Verification items for the finished model (mm, model axes). A direction names the side the tool comes from. Round coordinates to 2 decimals unless told otherwise and drop trailing zeros. Write each loop counter-clockwise with the first axis right and the second up, starting at its lowest first coordinate (ties: lowest second). Pieces come first, ordered by that corner, then holes.
Solid Edge part; units mm, degrees
sketch "Sketch1" plane through (0, 0, 0) normal (0, 0, 1) x (1, 0, 0)
  line L0 (0, 0) -> (12.7, 0)
  line L1 (0, 0) -> (-5.8373, 4.898)
sketch "Sketch2" plane through (12.7, 0, 0) normal (1, 0, 0) x (0, 1, 0)
  line L0 (1.5875, -1.5875) -> (1.5875, 1.5875)
  line L1 (1.5875, 1.5875) -> (-1.5875, 1.5875)
  line L2 (-1.5875, 1.5875) -> (-1.5875, -1.5875)
  line L3 (-1.5875, -1.5875) -> (1.5875, -1.5875)
sweep "SweptProtrusion_1" add profiles "Sketch2" path "Sketch1"
sketch "Sketch3" plane through (0, 0, 0) normal (0, 0, 1) x (1, 0, 0)
  line L0 (0, 0) -> (12.7, 0)
  line L1 (0, 0) -> (-6.5307, -7.783)
sketch "Sketch4" plane through (12.7, 0, 0) normal (1, 0, 0) x (0, 1, 0)
  line L0 (-1.5875, -1.5875) -> (1.5875, -1.5875)
  line L1 (1.5875, -1.5875) -> (1.5875, 1.5875)
  line L2 (1.5875, 1.5875) -> (-1.5875, 1.5875)
  line L3 (-1.5875, 1.5875) -> (-1.5875, -1.5875)
sweep "SweptProtrusion_2" add profiles "Sketch4" path "Sketch3"
sketch "Sketch5" plane through (-2.2223, 2.052, 1.5875) normal (0, 0, 1) x (1, 0, 0)
  circle A0 centre (2.2223, -2.052) radius 0.3969
extrude "Cutout1" cut sketch "Sketch5" against normal up to next
fillet "Round_1" radius 0.254 27 edges at (6.7201, -1.5875, 1.5875) (-2.2872, -5.1955, 1.5875) (-4.9917, -3.4791, 1.5875) (-4.5471, 1.7431, 1.5875) (-2.1195, 3.8508, 1.5875) (6.6389, 1.5875, 1.5875) (12.7, 0, 1.5875) (12.7, 0, -1.5875) (12.7, -1.5875, 0) (12.7, 1.5875, 0) (6.7201, -1.5875, -1.5875) (0.7403, -1.5875, 0) (-2.2872, -5.1955, -1.5875) (-6.5307, -7.783, 1.5875) (-5.3146, -8.8034, 0) (-6.5307, -7.783, -1.5875) (-7.7468, -6.7626, 0) (-2.2365, -0.1957, 0) (-4.9917, -3.4791, -1.5875) (-4.5471, 1.7431, -1.5875) (-6.8577, 3.6819, 0) (-5.8373, 4.898, 1.5875) (-4.8168, 6.1141, 0) (-5.8373, 4.898, -1.5875) (0.5778, 1.5875, 0) (6.6389, 1.5875, -1.5875) (-2.1195, 3.8508, -1.5875)
Q1. Tool access check on faces 4 (the cylindrical face through (-4.47, 1.77, -1.51)), 5 (the flat face through (7, 1.588, 0)), 6 (the cylindrical face through (-4.468, 1.777, 1.515)). Record the directions out of +Z, -Z, +X, -X, +Y, -Y that give a thin tool (end or side, any length) a straight path to the whole face; none if there is none.
Recorded:
face 4: -Z, -X
face 5: +Z, -Z, +X, +Y
face 6: +Z, -X
Q2. Sectioned sample at A-A (z = 0.4). Enter the section's corners in (x, y), plus the area to 3 significant figures.
Recorded:
outline: (-7.58, -6.57) arc R0.25 ccw to (-7.55, -6.93) - (-5.51, -8.64) arc R0.25 ccw to (-5.15, -8.61) - (0.66, -1.68) arc R0.25 cw to (0.86, -1.59) - (12.45, -1.59) arc R0.25 ccw to (12.7, -1.33) - (12.7, 1.33) arc R0.25 ccw to (12.45, 1.59) - (0.67, 1.59) arc R0.25 cw to (0.51, 1.65) - (-4.62, 5.95) arc R0.25 ccw to (-4.98, 5.92) - (-6.69, 3.88) arc R0.25 ccw to (-6.66, 3.52) - (-2.43, -0.03) arc R0.25 cw to (-2.4, -0.39) - close; hole circle Ø0.79 at (0, 0)
area: 91.6 mm2
Q3. Material ranges on line 1 along Y through (x, z) = (-4.25, -0.75); line 2 along Y through (x, z) = (5.5, -1.05); line 3 along Y through (x, z) = (-5, -0.8), recorded low to high.
Recorded:
line 1: y = -7.53 to -2.6, 1.49 to 5.64
line 2: y = -1.59 to 1.59
line 3: y = -8.43 to -3.49, 2.12 to 5.9
Q4. Release check for a two-part mould opening along Y. For faces 1 (the flat face through (-5.85, 4.88, 0.02)), 2 (the cylindrical face through (-4.9, -3.48, 1.51)), 3 (the flat face through (-6.545, -7.771, -0.019)) record: released by +Y, released by -Y, zero draft, split by the parting line, or undercut.
Recorded:
face 1: released by +Y
face 2: undercut
face 3: released by -Y
Q5. Sectioned sample at B-B (x = 5.75). Enter the section's corners in (y, z).
Recorded:
outline: (-1.59, -1.33) arc R0.25 ccw to (-1.33, -1.59) - (1.33, -1.59) arc R0.25 ccw to (1.59, -1.33) - (1.59, 1.33) arc R0.25 ccw to (1.33, 1.59) - (-1.33, 1.59) arc R0.25 ccw to (-1.59, 1.33) - close
